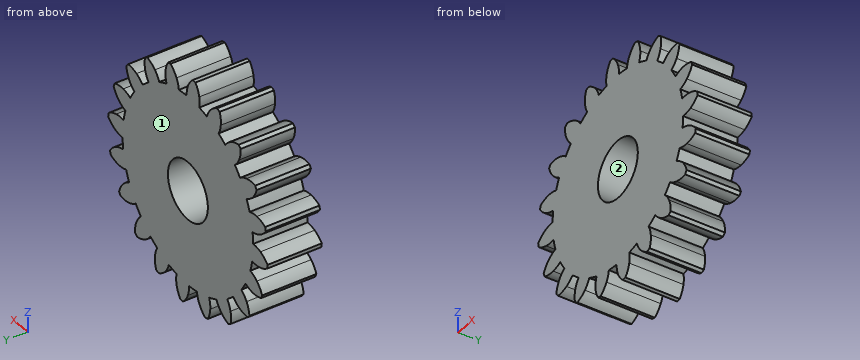
from build123d import *

# Parameters (mm, degrees)
F1_DEPTH = 2.8
F2_COUNT = 20
F2_ANGLE = 342
F3_R     = 1.5
F4_DEPTH = 2.8


with BuildPart() as f1:
    # F0 (on Front) → F1 (new body)
    with BuildSketch(Plane.XZ):
        with BuildLine():
            ThreePointArc((-0.856629721, 4.8346960112), (-0.38523416, 4.8948641086), (0.0897701035, 4.9091792928))
            ThreePointArc((0.0897701035, 4.9091792928), (0.0734017823, 5.1867797393), (0, 5.455))
            ThreePointArc((0, 5.455), (-0.1537545483, 5.7437546233), (-0.3707884455, 5.9885320345))
            ThreePointArc((-0.3707884455, 5.9885320345), (-0.4707851627, 5.9818926646), (-0.5705893808, 5.9728073599))
            ThreePointArc((-0.5705893808, 5.9728073599), (-0.7466596071, 5.6970919831), (-0.8533500068, 5.3878398979))
            ThreePointArc((-0.8533500068, 5.3878398979), (-0.8838891984, 5.1114393052), (-0.856629721, 4.8346960112))
        make_face()
        with BuildLine():
            ThreePointArc((-0.856629721, 4.8346960112), (-3.1545243754, -3.7625889976), (4.91, 0))
            ThreePointArc((4.91, 0), (3.5034890615, 3.4400093599), (0.0897701035, 4.9091792928))
            ThreePointArc((0.0897701035, 4.9091792928), (-0.38523416, 4.8948641086), (-0.856629721, 4.8346960112))
        make_face()
    extrude(amount=F1_DEPTH)

    # F2: F1 ×20 about axis
    f2_axis = Axis((0, 0, 0), (0, 1, 0))


with BuildPart() as f1_1:
    add(f1.part)
    for i in range(1, F2_COUNT):
        add(f1.part.rotate(f2_axis, i * F2_ANGLE / (F2_COUNT - 1)))

    # F3 (on face) → F4 (cut)
    with BuildSketch(Plane.XZ):
        Circle(F3_R)
    extrude(amount=F4_DEPTH, mode=Mode.SUBTRACT)


solid = f1_1.part
Source: CAD feature listing. Evaluate the final solid. Frame: model axes, mm. Face numbers are marked on the shaded views. Give positions to 0.01 mm unless a question says otherwise; leave off trailing zeros. Write each loop counter-clockwise with the first axis right and the second up, starting at its lowest first coordinate (ties: lowest second). Pieces come first, ordered by that corner, then holes. Notation, with made-up numbers: (29, 6) -> (70, 6) arc R29 cw to (70, 44) -> close; hole circle Ø8 at (74, 69). An arc over 180 degrees is marked (long way). Write item = value, one per line.
Q1. Line query: line 1 (Z direction, x = 5.25, y = -0.1); line 2 (X direction, y = -1.5, z = 3.75); line 3 (Z direction, x = 0.5, y = -2.6). Output: solid intervals per line, ascending. Write a range as from..to.
Here are the results:
line_1 = -1.68..-0.78, -0.06..0.88, 1.74..2.46
line_2 = -3.8..3.17, 3.66..4.62
line_3 = -5.98..-1.41, 1.41..4.88
Q2. Cut plane A-A on z = -2. Return loops of the section in (x, y), then the cut area to 3 significant figures.
Here are the results:
outline = (-5.47, -2.8) -> (4.48, -2.8) -> (4.48, 0) -> (-5.47, 0) -> close
area = 27.9 mm²
Q3. First-contact query: pin 1 (1 mm diameter, centred on y = -1, z = 2.5, fed in from -X); pin 2 (5 mm diameter, centred on x = 0, z = 0, fed in from +Y); pin 3 (1 mm diameter, centred on x = -2, y = -0.5, fed in from +Z); pin 4 (1.5 mm diameter, centred on y = -1, z = 2, fed in from -X). Flat tips, straight axial feed; report the tip coordinate or a pass-through.
Here are the results:
pin_1 = -5.15
pin_2 = 0
pin_3 = 5.58
pin_4 = -5.86
Q4. Mould query, pull axis X, two halves, no side actions, for the marked faces 1 and 2. Classes: +X half, -X half, draft (parallel to the pull), parting line (faces both ways), or undercut.
Here are the results:
face_1 = draft
face_2 = undercut
